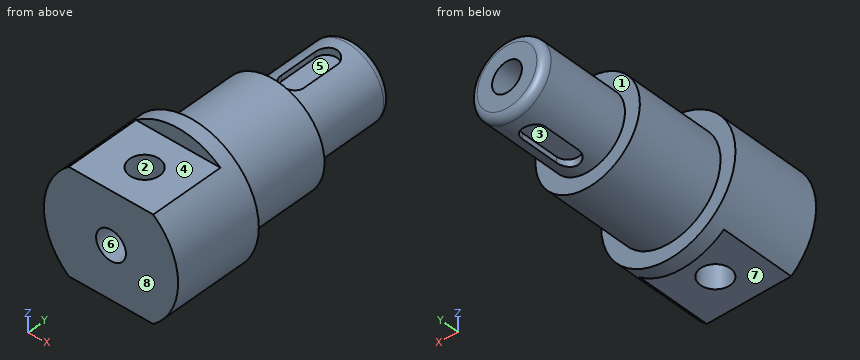
```python
from build123d import *

# Parameters (mm, degrees)
CUT_EXTRUDE2_DEPTH      = 45.09081537
CUT_EXTRUDE2_DEPTH_BACK = 45.09081537
SKETCH2_R               = 4
CUT_EXTRUDE3_START      = -14
SKETCH2_4_W             = 30
SKETCH2_4_H             = 25.460379871
SKETCH2_4_R             = 4
CUT_EXTRUDE3_DEPTH      = 31.090815533
CUT_EXTRUDE4_START      = 14
SKETCH2_5_W             = 30
SKETCH2_5_H             = 25.460379871
SKETCH2_5_R             = 4
CUT_EXTRUDE4_DEPTH      = 31.090815533
CUT_EXTRUDE5_START      = -8
CUT_EXTRUDE5_DEPTH      = 10
CUT_EXTRUDE6_START      = 18
CUT_EXTRUDE6_DEPTH      = 10


with BuildPart() as part:
    # Sketch1 → Revolve1 (revolve)
    with BuildSketch(Plane.XY, mode=Mode.PRIVATE) as revolve1_sk:
        with BuildLine():
            Line((18, -36), (18, -12))
            Line((18, -12), (14, -12))
            Line((14, -12), (14, 12))
            Line((14, 12), (10, 12))
            Line((10, 12), (10, 34))
            ThreePointArc((10, 34), (9.414213562, 35.414213562), (8, 36))
            Line((8, 36), (4, 36))
            Line((4, 36), (4, -36))
            Line((4, -36), (18, -36))
        make_face()
    revolve(revolve1_sk.sketch.rotate(Axis((0, -36, 0), (0, 1, 0)), 90), axis=Axis((0, -36, 0), (0, 1, 0)))

    # Sketch2 → Cut-Extrude2 (cut, two sides: drawn at the far end of the back side and taken through both)
    with BuildSketch(Plane.XY.offset(-CUT_EXTRUDE2_DEPTH_BACK)):
        with Locations(Location((0, -26, 0), (0, 0, 270))):
            Circle(SKETCH2_R)
    extrude(amount=CUT_EXTRUDE2_DEPTH + CUT_EXTRUDE2_DEPTH_BACK, mode=Mode.SUBTRACT)

    # Sketch2_4 → Cut-Extrude3 (cut, through all)
    with BuildSketch(Plane.XY.offset(CUT_EXTRUDE3_START)):
        with Locations((0, -28.730189936)):
            Rectangle(SKETCH2_4_W, SKETCH2_4_H)
        with Locations((0, -26)):
            Circle(SKETCH2_4_R, mode=Mode.SUBTRACT)
    extrude(amount=-CUT_EXTRUDE3_DEPTH, mode=Mode.SUBTRACT)

    # Sketch2_5 → Cut-Extrude4 (cut, through all)
    with BuildSketch(Plane.XY.offset(CUT_EXTRUDE4_START)):
        with Locations((0, -28.730189936)):
            Rectangle(SKETCH2_5_W, SKETCH2_5_H)
        with Locations((0, -26)):
            Circle(SKETCH2_5_R, mode=Mode.SUBTRACT)
    extrude(amount=CUT_EXTRUDE4_DEPTH, mode=Mode.SUBTRACT)

    # Sketch4 → Cut-Extrude5 (cut)
    with BuildSketch(Plane.XY.offset(CUT_EXTRUDE5_START)):
        with BuildLine():
            Line((3, 28), (3, 18))
            ThreePointArc((3, 18), (0, 15), (-3, 18))
            Line((-3, 18), (-3, 28))
            ThreePointArc((-3, 28), (0, 31), (3, 28))
        make_face()
    extrude(amount=-CUT_EXTRUDE5_DEPTH, mode=Mode.SUBTRACT)

    # Sketch4_2 → Cut-Extrude6 (cut)
    with BuildSketch(Plane.XY.offset(CUT_EXTRUDE6_START)):
        with BuildLine():
            Line((3, 28), (3, 18))
            ThreePointArc((3, 18), (0, 15), (-3, 18))
            Line((-3, 18), (-3, 28))
            ThreePointArc((-3, 28), (0, 31), (3, 28))
        make_face()
    extrude(amount=-CUT_EXTRUDE6_DEPTH, mode=Mode.SUBTRACT)


solid = part.part
```
CAD build for the part. Positions are in the model's coordinates, mm. Face numbers are marked on the shaded views. A direction names the side the tool comes from. Coordinates: 2 decimals unless noted, no trailing zeros. Order: outer loops, then holes, each group sorted by start corner. A loop starts at its lowest first (then second) coordinate and runs counter-clockwise, first axis right, second up. Notation, with made-up numbers: (-15, -18.5) -> (29, -18.5) arc R24 ccw to (29, 3.5) -> close; hole circle Ø3 at (35, 52.5). An arc over 180 degrees is marked (long way). Use one line per item in the form item = value. Start each with the question number.
1) Band-saw the part on B-B on x = 0. State how many separate pieces and enclosed holes the cut face has, then the cut area to 3 significant figures.
2) Drill centre lines: L1, parallel to X at y = -33.5, z = 0; L2, parallel to Y at x = 0, z = 11; L3, parallel to Y at x = 1, z = 9. Where is each one in solid material? Low to high. Write a range as [from, to].
3) Band-saw the part on C-C on y = -15. Give the cut face in (x, z).
4) Band-saw the part on A-A on y = 11. Give the cut face in (x, z), then the cut area to 3 significant figures.
5) Pull direction Z, two halves, no side cores. Call the marked faces 6, 7 and 8: +Z half, -Z half, draft (parallel to the pull), parting line (faces both ways), or undercut.
6) Drop flat-ended pins along their axis: pin 1 (10.5 mm diameter, centred on x = 0, y = -26, fed in from -Z); pin 2 (3 mm diameter, centred on x = -2, z = -16, fed in from -Y); pin 3 (1.8 mm diameter, centred on x = 1, y = 26.5, fed in from -Z). Give the stop position or say it passes through.
7) Tool access for the marked faces 1, 2, 3, 4 and 5: list every direction of +Z, -Z, +X, -X, +Y, -Y with a clear straight run to the whole face (end or side of a thin tool).
Entries:
q1.separate_pieces = 4
q1.enclosed_holes = 0
q1.area = 1,050 mm2
q2.L1 = [-18, -4], [4, 18]
q2.L2 = [-36, -30], [-22, 12]
q2.L3 = [-36, -29.87], [-22.13, 15.17], [30.83, 35.7]
q3.outline = circle Ø36 at (0, 0); hole circle Ø8 at (0, 0)
q4.outline = circle Ø28 at (0, 0); hole circle Ø8 at (0, 0)
q4.area = 565 mm2
q5.face_6 = undercut
q5.face_7 = -Z half
q5.face_8 = draft
q6.pin_1 = -14
q6.pin_2 = -16
q6.pin_3 = -8
q7.face_1 = +Y
q7.face_2 = +Z, -Z
q7.face_3 = -Z
q7.face_4 = +Z, +X, -X, -Y
q7.face_5 = +Z
